Could you check a few things on this model? Use its own coordinates, in mm. Round coordinates to 2 decimals unless told otherwise and drop trailing zeros. Loops run counter-clockwise (first coordinate to the right, second up) from the corner with the lowest first, then second, coordinate; pieces in that order, holes last. Notation, with made-up numbers: (-35, 9) - (16, 9) arc R30 cw to (16, 45) - close; hole circle Ø11 at (62.5, 35.25). An arc over 180 degrees is marked (long way). Use one line per item in the form item = value.
```python
from build123d import *

# Parameters (mm, degrees)
CROQUIS1_R              = 2.5
CROQUIS1_W              = 5.5
CROQUIS1_H              = 20
SALIENTE_EXTRUIR2_DEPTH = 5.5


with BuildPart() as part:
    # Croquis1 → Saliente-Extruir2 (new body)
    with BuildSketch(Plane.XY):
        Polygon((-291.621999317, -23.071413697), (101.378000683, -23.071413697), (101.378000683, -17.571413697), (209.378000683, -17.571413697), (209.378000683, -23.071413697), (317.378000683, -23.071413697), (317.378000683, -17.571413697), (425.378000683, -17.571413697), (425.378000683, -23.071413697), (533.378000683, -23.071413697), (533.378000683, -17.571413697), (641.378000683, -17.571413697), (641.378000683, 326.928586303), (-291.621999317, 326.928586303), align=None)
        with Locations((-195.121999317, 285.627487196)):
            Circle(CROQUIS1_R, mode=Mode.SUBTRACT)
        with Locations((-95.121999317, 285.627487196)):
            Circle(CROQUIS1_R, mode=Mode.SUBTRACT)
        with Locations((4.878000683, 285.627487196)):
            Circle(CROQUIS1_R, mode=Mode.SUBTRACT)
        with Locations((-238.871999317, 10.407487196)):
            Rectangle(CROQUIS1_W, CROQUIS1_H, mode=Mode.SUBTRACT)
        with Locations((48.628000683, 10.407487196)):
            Rectangle(CROQUIS1_W, CROQUIS1_H, mode=Mode.SUBTRACT)
        with Locations((-238.871999317, 40.407487196)):
            Rectangle(CROQUIS1_W, CROQUIS1_H, mode=Mode.SUBTRACT)
        with Locations((48.628000683, 40.407487196)):
            Rectangle(CROQUIS1_W, CROQUIS1_H, mode=Mode.SUBTRACT)
        Polygon((576.378000683, 296.928586303), (566.378000683, 296.928586303), (566.378000683, 291.428586303), (586.378000683, 291.428586303), (586.378000683, 296.928586303), align=None, mode=Mode.SUBTRACT)
        with Locations((104.128000683, 19.428586303)):
            Rectangle(CROQUIS1_W, CROQUIS1_H, mode=Mode.SUBTRACT)
    extrude(amount=SALIENTE_EXTRUIR2_DEPTH)


solid = part.part
```
1. If we section it at A-A, the plane x = 188.5: Write out the boundary of the cut face in (y, z), plus the area to 3 significant figures.
Solution:
outline = (-17.57, 0) - (326.93, 0) - (326.93, 5.5) - (-17.57, 5.5) - close
area = 1,890 mm^2
2. Please list where these lines run through material, in increasing order: line 1 along X through (y, z) = (50, 3.25); line 2 along X through (y, z) = (14, 3.75); line 3 along X through (y, z) = (295, 4.05).
Solution:
line_1 = -291.62 to -241.62, -236.12 to 45.88, 51.38 to 641.38
line_2 = -291.62 to -241.62, -236.12 to 45.88, 51.38 to 101.38, 106.88 to 641.38
line_3 = -291.62 to 566.38, 586.38 to 641.38
3. For P1, Ø1.6, axis at x = 585, z = 2.5, coming from the -Y side; P2, Ø6.5, axis at x = 4.88, y = 285.63, coming from the -Z side; P3, Ø1.6, axis at y = -19.5, z = 2, coming from the +X side, each with a flat end and sliding along its axis, tell me the tip position at first contact or that it passes through.
Solution:
P1 = -17.57
P2 = 0
P3 = 533.38
